```python
from build123d import *
from build123d.topology import SkipClean

# Parameters (mm, degrees)
SKETCH1_R         = 6
EXTRUDE1_DEPTH    = 21.5
EXTRUDE2_REACH    = 33.875
CIRPATTERN1_COUNT = 8


with BuildPart() as part:
    # Sketch1 → Extrude1 (new body)
    with BuildSketch(Plane.XY):
        with BuildLine():
            ThreePointArc((3.535156209, 14.285110262), (0, 16.64), (-3.535156209, 14.285110262))
            ThreePointArc((-3.535156209, 14.285110262), (-7.848885271, 7.848885271), (-14.285110262, 3.535156209))
            ThreePointArc((-14.285110262, 3.535156209), (-16.64, 0), (-14.285110262, -3.535156209))
            ThreePointArc((-14.285110262, -3.535156209), (-7.848885271, -7.848885271), (-3.535156209, -14.285110262))
            ThreePointArc((-3.535156209, -14.285110262), (0, -16.64), (3.535156209, -14.285110262))
            ThreePointArc((3.535156209, -14.285110262), (7.848885271, -7.848885271), (14.285110262, -3.535156209))
            ThreePointArc((14.285110262, -3.535156209), (16.64, 0), (14.285110262, 3.535156209))
            ThreePointArc((14.285110262, 3.535156209), (7.848885271, 7.848885271), (3.535156209, 14.285110262))
        make_face()
        Circle(SKETCH1_R, mode=Mode.SUBTRACT)
    extrude(amount=EXTRUDE1_DEPTH)

    # Sketch4 → Cut-Revolve1 (revolve, cut)
    with BuildSketch(Plane(origin=(0, 0, 0), x_dir=(0, 0, -1), z_dir=(1, 0, 0)), mode=Mode.PRIVATE) as cut_revolve1_sk:
        Polygon((0, 0), (-21.5, 0), (-21.5, 6.05), (-7.2, 6.05), (-5, 8.25), (0, 8.25), align=None)
    revolve(cut_revolve1_sk.sketch.rotate(Axis((0, 0, 0), (0, 0, 1)), 90), axis=Axis((0, 0, 0), (0, 0, 1)), mode=Mode.SUBTRACT)

    # Sketch2 → Extrude2 (cut, up to next)
    with BuildSketch(Plane(origin=(0, 0, 0), x_dir=(-1, 0, 0), z_dir=(0, 0, -1)), mode=Mode.PRIVATE) as extrude2_sk1:
        with BuildLine():
            ThreePointArc((0.75, 8.215838363), (0, 8.25), (-0.75, 8.215838363))
            ThreePointArc((-0.75, 8.215838363), (-1.133672744, 7.067180744), (-1.4, 5.885787968))
            ThreePointArc((-1.4, 5.885787968), (0, 6.05), (1.4, 5.885787968))
            ThreePointArc((1.4, 5.885787968), (1.133672744, 7.067180744), (0.75, 8.215838363))
        make_face()
    extrude2_tool1 = extrude(extrude2_sk1.sketch, amount=-EXTRUDE2_REACH, mode=Mode.PRIVATE) & part.part
    extrude2 = extrude2_tool1.solids().sort_by_distance((0, 7.008505, 0))[0]
    add(extrude2, mode=Mode.SUBTRACT)

    # CirPattern1: Extrude2 ×8 about axis
    with SkipClean():  # the faces are left unmerged after this step: merging them gives an invalid solid
        cirpattern1_axis = Axis((0, 0, 0), (0, 0, 1))
        for i in range(1, CIRPATTERN1_COUNT):
            add(extrude2.rotate(cirpattern1_axis, i * 360 / CIRPATTERN1_COUNT), mode=Mode.SUBTRACT)


solid = part.part
```
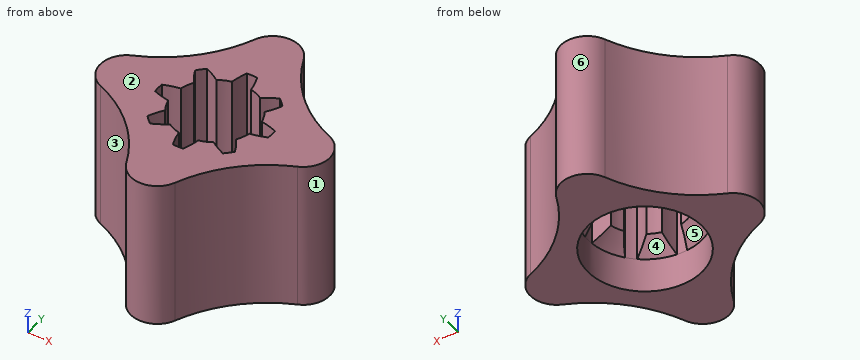
Model file for the job. Use its own axes, mm. Face numbers are marked on the shaded views. A direction names the side the tool comes from. Round coordinates to 2 decimals unless told otherwise and drop trailing zeros. Write each loop counter-clockwise with the first axis right and the second up, starting at its lowest first coordinate (ties: lowest second). Pieces come first, ordered by that corner, then holes. Notation, with made-up numbers: M -40,0.25 L -19,0.25 A29 ccw -19,32.25 Z; hole C 85,36.25 d1. An arc over 180 degrees is marked long. Put each result on its own line as item: value.
Item 1: Probe L1, parallel to Y at x = 5.5, z = 8.25; L2, parallel to Y at x = -6, z = 9; L3, parallel to Y at x = 0, z = 1.55. List the from-to ranges inside material, lowest first. Write a range as from..to.
Responses:
L1: -10.68..-6.15, -3.69..-2.52, 2.52..3.69, 6.15..10.68
L2: -9.98..-5.66, -4.57..-1.38, 1.38..4.57, 5.66..9.98
L3: -16.64..-8.25, 8.25..16.64
Item 2: Cut at C-C (x = -13). List the corners of the cut face in (y, z), and give its area (3 significant figures).
Responses:
outline: M -4.13,0 L 4.13,0 L 4.13,21.5 L -4.13,21.5 Z
area: 177 mm²
Item 3: Tool access for the marked faces 5 and 6: list every direction of +Z, -Z, +X, -X, +Y, -Y with a clear straight run to the whole face (end or side of a thin tool).
Responses:
face 5: -Z
face 6: +Z, -Z, +Y
Item 4: Mould opens along X. For the marked faces 1, 2, 3 and 4 say: +X half, -X half, draft (parallel to the pull), parting line (faces both ways), or undercut.
Responses:
face 1: +X half
face 2: draft
face 3: -X half
face 4: undercut
Item 5: Cut at D-D (x = 11). List the corners of the cut face in (y, z), and give its area (3 significant figures).
Responses:
outline: M -5.28,0 L 5.28,0 L 5.28,21.5 L -5.28,21.5 Z
area: 227 mm²
Item 6: Flat gauge pins, fed straight in: P1, Ø8, axis at y = -7.5, z = 5.5, coming from the -X side; P2, Ø8, axis at y = -9.5, z = 14.5, coming from the -X side; P3, Ø10, axis at x = 0, y = 0, coming from the +Z side; P4, Ø12, axis at y = 10.5, z = 5.5, coming from the -X side. Where does each tip first touch, or does it go through?
Responses:
P1: x = -14.37
P2: x = -10.68
P3: through
P4: x = -12.29
Item 7: Cut at A-A (y = 0). List the corners of the cut face in (x, z).
Responses:
outline: M -16.64,0 L -8.25,0 L -8.25,21.5 L -16.64,21.5 Z; M 8.25,0 L 16.64,0 L 16.64,21.5 L 8.25,21.5 Z
